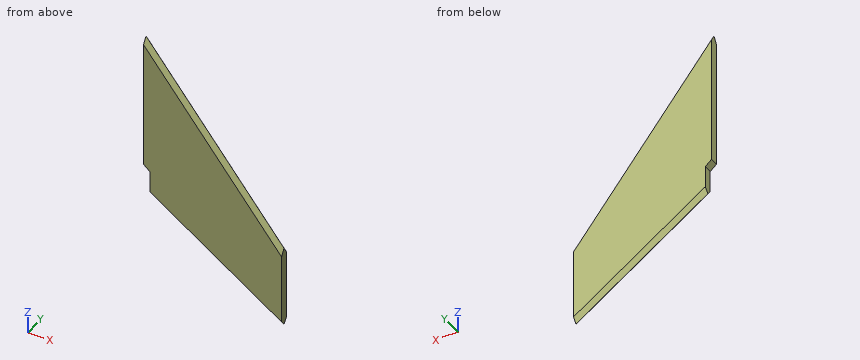
```python
from build123d import *

# Parameters (mm, degrees)
F1_DEPTH = 3
F2_SIZE  = 1.49999
F4_DEPTH = 4


# Not quite as in the source:
# - a fillet or chamfer is up to 0.001 mm smaller than in the source, because OpenCascade refuses the exact size


with BuildPart() as f1:
    # F0 (on Front) → F1 (new body)
    with BuildSketch(Plane.XZ):
        Polygon((0, 60), (0, 0), (50, -34.25), (50, -4.25), align=None)
    extrude(amount=F1_DEPTH)

    # F2 (size 1.5 in the source; OpenCascade refuses exactly that, so slightly less here)
    f2_edges = [f1.edges().sort_by_distance(p)[0] for p in [
        (25, -3, 27.875),
        (25, 0, 27.875),
        (25, -3, -17.125),
        (25, 0, -17.125),
    ]]
    chamfer(f2_edges, length=F2_SIZE)

    # F3 (on Front) → F4 (cut, symmetric)
    with BuildSketch(Plane.XZ):
        Polygon((2.25, 8.25), (0, 10.25), (0, -5), (2.25, -5), align=None)
    extrude(amount=F4_DEPTH, both=True, mode=Mode.SUBTRACT)


solid = f1.part
```
Verification items for the finished model (mm, model axes). Coordinates: 2 decimals unless noted, no trailing zeros. Order: outer loops, then holes, each group sorted by start corner. A loop starts at its lowest first (then second) coordinate and runs counter-clockwise, first axis right, second up. Notation, with made-up numbers: (22, 6) -> (48, 6) arc R30 ccw to (48, 34) -> close; hole circle Ø4 at (78, -16). An arc over 180 degrees is marked (long way). Put each result on its own line as item: value. Start each with the question number.
1) Go/stop test with flat-tipped pins: pin 1 (1.5 mm diameter, centred on y = -1, z = 3, fed in from -X); pin 2 (1.5 mm diameter, centred on y = -0.5, z = 7, fed in from +X); pin 3 (12 mm diameter, centred on x = 33.5, z = 18, fed in from +Y). Record where each tip stops, or that it passes through.
2) Cross-section at C-C (y = -0.55). Enter the section's corners in (x, z), plus the area to 3 significant figures.
3) Material ranges on L1, parallel to X at y = -2.4, z = 30; L2, parallel to Z at x = 3.5, y = -1.65; L3, parallel to Z at x = 2, y = -0.4, recorded low to high.
Geometry check:
1. pin 1: stops at x = 2.25
1. pin 2: stops at x = 41.09
1. pin 3: stops at y = 0
2. outline: (0, 10.25) -> (2.25, 8.25) -> (2.25, -0.39) -> (50, -33.1) -> (50, -5.8) -> (0, 58.45) -> close
2. area: 2,100 mm^2
3. L1: x = 0 to 22.21
3. L2: z = -2.22 to 55.26
3. L3: z = 8.47 to 55.64
